Read the model definition and answer for the solid it produces. Units are mm, in the model's axes. Give positions to 0.01 mm unless a question says otherwise; leave off trailing zeros. Loops run counter-clockwise (first coordinate to the right, second up) from the corner with the lowest first, then second, coordinate; pieces in that order, holes last. Notation, with made-up numbers: (-5.75, 33.25) - (37.25, 33.25) arc R31 cw to (37.25, 65.25) - close; hole circle Ø7 at (51, 80.25). An arc over 180 degrees is marked (long way). Use a Markdown table: item, result. Add a question column.
Item 1: This flat-tipped pin is pushed along its axis until it touches: P1, Ø1.4, axis at x = 7.5, z = -143.15, coming from the +Y side. Where does it stop, or does it pass through?
Item 2: A cutting plane is placed at B-B (z = -57.15). Determine the outline of the cut face in (x, y) (3 decimals), plus the area to 3 significant figures.
Item 3: For a pull along X with two mould halves and no side action, classify faces 1 (the face through (27.684, 1.541, -34.241)), 2 (the face through (0, 2, -73)), 3 (the face through (22.463, 1.541, -60.98)), 4 (the face through (42, 2, 0)) as +X half, -X half, draft (parallel to the pull), parting line (faces both ways), or undercut.
Item 4: Consider probe 1 along X at (y, z) = (1.15, -57.15); probe 2 along X at (y, z) = (1.4, -78.15); probe 3 along X at (y, z) = (2.1, -123.15). Determine where each line is inside the solid, lowest interval first. Write a range as [from, to].
Item 5: A cutting plane is placed at A-A (z = -6.35). Determine the outline of the cut face in (x, y) (3 decimals).
Item 6: A cutting plane is placed at C-C (y = 1.7). Give the number of separate pieces and of enclosed holes in the cut face, plus the area to 3 significant figures.
from build123d import *

# Parameters (mm, degrees)
SKETCH1_W           = 85
SKETCH1_H           = 147.15
SKETCH1_R           = 4.826
SKETCH1_R_2         = 3.38
SKETCH1_R_3         = 0.889
BOSS_EXTRUDE1_DEPTH = 3.125


with BuildPart() as part:
    # Sketch1 → Boss-Extrude1 (new body)
    with BuildSketch(Plane(origin=(0, 0, 0), x_dir=(1, 0, 0), z_dir=(0, 1, 0))):
        with Locations((42.5, 73.575)):
            Rectangle(SKETCH1_W, SKETCH1_H)
        with Locations(Location((25.4, 57.15, 0), (0, 0, 270))):
            Circle(SKETCH1_R, mode=Mode.SUBTRACT)
        with Locations(Location((25.4, 31.75, 0), (0, 0, 270))):
            Circle(SKETCH1_R_2, mode=Mode.SUBTRACT)
        with Locations(Location((25.4, 6.35, 0), (0, 0, 270))):
            Circle(SKETCH1_R_2, mode=Mode.SUBTRACT)
        with Locations(Location((50.8, 57.15, 0), (0, 0, 270))):
            Circle(SKETCH1_R_2, mode=Mode.SUBTRACT)
        with Locations(Location((7.5, 143.15, 0), (0, 0, 270))):
            Circle(SKETCH1_R_3, mode=Mode.SUBTRACT)
        with Locations(Location((77.5, 143.15, 0), (0, 0, 270))):
            Circle(SKETCH1_R_3, mode=Mode.SUBTRACT)
        with Locations(Location((77.5, 78.15, 0), (0, 0, 270))):
            Circle(SKETCH1_R_3, mode=Mode.SUBTRACT)
        with Locations(Location((7.5, 78.15, 0), (0, 0, 270))):
            Circle(SKETCH1_R_3, mode=Mode.SUBTRACT)
        with Locations(Location((12.7, 123.15, 0), (0, 0, 270))):
            Circle(SKETCH1_R_3, mode=Mode.SUBTRACT)
        with Locations(Location((25.7, 90.15, 0), (0, 0, 270))):
            Circle(SKETCH1_R_3, mode=Mode.SUBTRACT)
        with Locations(Location((25.7, 123.15, 0), (0, 0, 270))):
            Circle(SKETCH1_R_3, mode=Mode.SUBTRACT)
        with Locations(Location((12.7, 90.15, 0), (0, 0, 270))):
            Circle(SKETCH1_R_3, mode=Mode.SUBTRACT)
        with Locations(Location((38.1, 123.15, 0), (0, 0, 270))):
            Circle(SKETCH1_R_3, mode=Mode.SUBTRACT)
        with Locations(Location((51.1, 123.15, 0), (0, 0, 270))):
            Circle(SKETCH1_R_3, mode=Mode.SUBTRACT)
        with Locations(Location((51.1, 90.15, 0), (0, 0, 270))):
            Circle(SKETCH1_R_3, mode=Mode.SUBTRACT)
        with Locations(Location((38.1, 90.15, 0), (0, 0, 270))):
            Circle(SKETCH1_R_3, mode=Mode.SUBTRACT)
    extrude(amount=BOSS_EXTRUDE1_DEPTH)


solid = part.part
Geometry says:
| question | item | result |
|---|---|---|
| 1 | P1 | through |
| 2 | outline | (0, 0) - (20.574, 0) - (20.574, 3.125) - (0, 3.125) - close; (30.226, 0) - (47.42, 0) - (47.42, 3.125) - (30.226, 3.125) - close; (54.18, 0) - (85, 0) - (85, 3.125) - (54.18, 3.125) - close |
| 2 | area | 214 mm² |
| 3 | face 1 | undercut |
| 3 | face 2 | -X half |
| 3 | face 3 | undercut |
| 3 | face 4 | draft |
| 4 | probe 1 | [0, 20.57], [30.23, 47.42], [54.18, 85] |
| 4 | probe 2 | [0, 6.61], [8.39, 76.61], [78.39, 85] |
| 4 | probe 3 | [0, 11.81], [13.59, 24.81], [26.59, 37.21], [38.99, 50.21], [51.99, 85] |
| 5 | outline | (0, 0) - (22.02, 0) - (22.02, 3.125) - (0, 3.125) - close; (28.78, 0) - (85, 0) - (85, 3.125) - (28.78, 3.125) - close |
| 6 | separate pieces | 1 |
| 6 | enclosed holes | 16 |
| 6 | area | 12,300 mm² |
